Design review of the part built by this model. Coordinates are the model's own, in mm. A direction names the side the tool comes from. Give positions to 0.01 mm unless a question says otherwise; leave off trailing zeros. Loops run counter-clockwise (first coordinate to the right, second up) from the corner with the lowest first, then second, coordinate; pieces in that order, holes last. Notation, with made-up numbers: M 82,86 L 99,86 A20 cw 99,123 Z; hole C 12,58.25 d11. An arc over 180 degrees is marked long. Use a Markdown table: item, result. Add a question column.
(1) For probe 1 along Z at (x, y) = (1.75, 10); probe 2 along Z at (x, y) = (7, 47.5); probe 3 along Z at (x, y) = (6, 44), list the stretches that pass through material, from the lowest coordinate up.
(2) Add section D-D, the plane x = 9. Give the boundary of the cut face in (y, z), then the cut area to 3 significant figures.
(3) Add section A-A, the plane x = 6. Give the boundary of the cut face in (y, z).
(4) Draft analysis for pull direction X (two halves, no side actions). For faces 4 (the face through (0, 33, 1)), 5 (the face through (11, 33.9, 1.5)), 6 (the face through (4.4, 26.2, 5.5)), 7 (the face through (6.1, 61, 0.5)), state which applies: pulls with the +X half, pulls with the -X half, needs draft (parallel to the pull), parting line crosses it, or undercut.
(5) Add section B-B, the plane y = 25. Give the boundary of the cut face in (x, z), then the cut area to 3 significant figures.
(6) For faces 1 (the face through (6, 47, 5)), 2 (the face through (1, 33.9, 1.5)), 3 (the face through (2, 32.9, 0.5)), list the 3-axis set-ups (+Z, -Z, +X, -X, +Y, -Y) from which the entire face can be reached by the end or side of a thin tool; tool diameter is ignored.
(7) Add section C-C, the plane z = 7.25. Give the boundary of the cut face in (x, y).
(8) Insertion check: pin 1 Ø1.1 at (y, z) = (44.5, 0.5) entering from -X; pin 2 Ø2 at (x, y) = (6, 50.5) entering from +Z; pin 3 Ø5 at (x, y) = (7, 46) entering from -Z; pin 4 Ø2 at (x, z) = (5.5, 5) entering from +Y. Each pin has a flat end and moves straight along its axis. Give the tip position at first contact, or say it passes through.
Autodesk Inventor part; units mm, degrees
ref_plane "YZ Plane" through (0, 0, 0) normal (1, 0, 0) x (0, 1, 0)
ref_plane "XZ Plane" through (0, 0, 0) normal (0, 1, 0) x (-1, 0, 0)
ref_plane "XY Plane" through (0, 0, 0) normal (0, 0, 1) x (1, 0, 0)
sketch "Sketch1" plane through (0, 0, 0) normal (0, 0, 1) x (1, 0, 0)
  line L0 (0, 0) -> (12, 0)
  line L1 (12, 0) -> (12, 65)
  line L2 (12, 65) -> (0, 65)
  line L3 (0, 65) -> (0, 0)
  dimension "d0" = 65
  dimension "d1" = 12
extrude "Extrusion1" add sketch "Sketch1" along normal blind 3
sketch "Sketch2" plane through (0, 0, 3) normal (0, 0, 1) x (1, 0, 0)
  circle A0 centre (6, 45) radius 2
  circle A1 centre (6, 25) radius 2
  line L0 (0, 65) -> (0, 0)
  line L1 (12, 0) -> (12, 65)
  line L2 (12, 65) -> (0, 65)
  dimension "d4" = 12
  dimension "d5" = 6
  dimension "d6" = 0
  dimension "d7" = 20
  dimension "d8" = 20
  dimension "d9" = 4
extrude "Extrusion2" add sketch "Sketch2" along normal blind 5
sketch "Sketch3" plane through (0, 65, 0) normal (0, 1, 0) x (1, 0, 0)
  line L0 (1, -2) -> (11, -2)
  line L1 (11, -2) -> (11, -1)
  line L2 (11, -1) -> (1, -1)
  line L3 (1, -1) -> (1, -2)
  line L4 (12, 0) -> (0, 0)
  line L5 (0, 0) -> (0, -3)
  line L6 (12, 0) -> (12, -3)
  dimension "d12" = 1
  dimension "d13" = 1
  dimension "d14" = 1
  dimension "d15" = 1
sketch "Sketch4" plane through (0, 0, 3) normal (0, 0, 1) x (1, 0, 0)
  line L0 (0, 0) -> (12, 0)
  line L1 (12, 65) -> (0, 65)
  dimension "d16" = 65
extrude "Extrusion3" cut sketch "Sketch3" against normal blind 63
sketch "Sketch5" plane through (0, 0, 0) normal (0, 0, -1) x (-1, 0, 0)
  point P0 (0, 0)
sketch "Sketch6" plane through (0, 0, 0) normal (0, 0, -1) x (-1, 0, 0)
  line L0 (-10, 61) -> (-2, 61)
  line L1 (-2, 61) -> (-2, 4)
  line L2 (-2, 4) -> (-10, 4)
  line L3 (-10, 4) -> (-10, 61)
  line L4 (0, 0) -> (-12, 0)
  line L5 (-12, 65) -> (0, 65)
  line L6 (0, 65) -> (0, 0)
  line L7 (-12, 0) -> (-12, 65)
  dimension "d19" = 4
  dimension "d20" = 4
  dimension "d21" = 2
  dimension "d22" = 2
extrude "Extrusion4" cut sketch "Sketch6" against normal up to surface (2 mm away) contours L0 L1 L2 L3
properties part number "covet cover"
Established:
| question | item | result |
|---|---|---|
| 1 | probe 1 | 0 to 1, 2 to 3 |
| 1 | probe 2 | 2 to 3 |
| 1 | probe 3 | 2 to 8 |
| 2 | outline | M 0,0 L 4,0 L 4,1 L 2,1 L 2,2 L 65,2 L 65,3 L 0,3 Z; M 61,0 L 65,0 L 65,1 L 61,1 Z |
| 2 | area | 75.0 mm^2 |
| 3 | outline | M 0,0 L 4,0 L 4,1 L 2,1 L 2,2 L 65,2 L 65,3 L 47,3 L 47,8 L 43,8 L 43,3 L 27,3 L 27,8 L 23,8 L 23,3 L 0,3 Z; M 61,0 L 65,0 L 65,1 L 61,1 Z |
| 4 | face 4 | pulls with the -X half |
| 4 | face 5 | undercut |
| 4 | face 6 | parting line crosses it |
| 4 | face 7 | undercut |
| 5 | outline | M 0,0 L 2,0 L 2,1 L 1,1 L 1,2 L 11,2 L 11,1 L 10,1 L 10,0 L 12,0 L 12,3 L 8,3 L 8,8 L 4,8 L 4,3 L 0,3 Z |
| 5 | area | 38.0 mm^2 |
| 6 | face 1 | +Z |
| 6 | face 2 | +Y |
| 6 | face 3 | -Z |
| 7 | outline | C 6,25 d4; C 6,45 d4 |
| 8 | pin 1 | x = 0 |
| 8 | pin 2 | z = 3 |
| 8 | pin 3 | z = 2 |
| 8 | pin 4 | y = 47 |
